from build123d import *

# Parameters (mm, degrees)
SKETCH1_W            = 170
SKETCH1_H            = 72
BOSS_EXTRUDE1_DEPTH  = 5
SKETCH2_R            = 5.5
SKETCH2_R_2          = 3.025
BOSS_EXTRUDE2_DEPTH  = 5
BOSS_EXTRUDE3_DEPTH  = 5
FILLET1_R            = 6
M4_CLEARANCE_HOLE1_D = 4.5


with BuildPart() as part:
    # Sketch1 → Boss-Extrude1 (new body)
    with BuildSketch(Plane.XY):
        Rectangle(SKETCH1_W, SKETCH1_H)
    extrude(amount=BOSS_EXTRUDE1_DEPTH)

    # Sketch2 → Boss-Extrude2 (add)
    # profile 1 of 6: a face of its own
    with BuildSketch(Plane.XY.offset(5)):
        with Locations((65, 25)):
            Circle(SKETCH2_R)
        with Locations((65, 25)):
            Circle(SKETCH2_R_2, mode=Mode.SUBTRACT)
    # profile 2 of 6: a face of its own
    with BuildSketch(Plane.XY.offset(5)):
        with Locations((8.25, 25)):
            Circle(SKETCH2_R)
        with Locations((8.25, 25)):
            Circle(SKETCH2_R_2, mode=Mode.SUBTRACT)
    # profile 3 of 6: a face of its own
    with BuildSketch(Plane.XY.offset(5)):
        with Locations((-65, 25)):
            Circle(SKETCH2_R)
        with Locations((-65, 25)):
            Circle(SKETCH2_R_2, mode=Mode.SUBTRACT)
    # profile 4 of 6: a face of its own
    with BuildSketch(Plane.XY.offset(5)):
        with Locations((-65, -25)):
            Circle(SKETCH2_R)
        with Locations((-65, -25)):
            Circle(SKETCH2_R_2, mode=Mode.SUBTRACT)
    # profile 5 of 6: a face of its own
    with BuildSketch(Plane.XY.offset(5)):
        with Locations((8.25, -25)):
            Circle(SKETCH2_R)
        with Locations((8.25, -25)):
            Circle(SKETCH2_R_2, mode=Mode.SUBTRACT)
    # profile 6 of 6: a face of its own
    with BuildSketch(Plane.XY.offset(5)):
        with Locations((65, -25)):
            Circle(SKETCH2_R)
        with Locations((65, -25)):
            Circle(SKETCH2_R_2, mode=Mode.SUBTRACT)
    extrude(amount=BOSS_EXTRUDE2_DEPTH)

    # Sketch3 → Boss-Extrude3 (add)
    with BuildSketch(Plane.XY.offset(5)):
        Polygon((-65, 51), (-85, 36), (-85, 51), align=None)
        Polygon((-65, 51), (-85, 36), (-65, 36), align=None)
        Polygon((65, -51), (85, -36), (65, -36), align=None)
        Polygon((85, -36), (85, -51), (65, -51), align=None)
    extrude(amount=-BOSS_EXTRUDE3_DEPTH)

    # Fillet1
    fillet1_edges = [part.edges().sort_by_distance(p)[0] for p in [
        (-85, 51, 2.5),
        (-65, 51, 2.5),
        (-65, 36, 2.5),
        (65, -51, 2.5),
        (65, -36, 2.5),
        (85, -51, 2.5),
        (-85, -36, 2.5),
        (85, 36, 2.5),
    ]]
    fillet(fillet1_edges, radius=FILLET1_R)

    # M4 Clearance Hole1 (through all)
    with Locations(Plane.XY.offset(5)):
        with Locations((-75, 43.5), (75, -43.5)):
            Hole(M4_CLEARANCE_HOLE1_D / 2)


solid = part.part
Part model, mm, in its own coordinate system. A direction names the side the tool comes from. Coordinates: 2 decimals unless noted, no trailing zeros. Write each loop counter-clockwise with the first axis right and the second up, starting at its lowest first coordinate (ties: lowest second). Pieces come first, ordered by that corner, then holes. Notation, with made-up numbers: (-26, 40.5) - (-10, 40.5) arc R18 cw to (-10, 64.5) - close; hole circle Ø9 at (49.25, -6). An arc over 180 degrees is marked (long way). Put each result on its own line as item: value.
1. Probe line 1 along Y through (x, z) = (8.25, 6.1) (3 decimals); line 2 along X through (y, z) = (30, 7); line 3 along Y through (x, z) = (67, 6.75). List the from-to ranges inside material, lowest first. Write a range as [from, to].
Final values:
line 1: y = [-30.5, -28.025], [-21.975, -19.5], [19.5, 21.975], [28.025, 30.5]
line 2: x = [-67.29, -62.71], [5.96, 10.54], [62.71, 67.29]
line 3: y = [-30.12, -27.27], [-22.73, -19.88], [19.88, 22.73], [27.27, 30.12]
2. Band-saw the part on C-C (x = 75). Write the cut outline in (y, z).
Final values:
outline: (-51, 0) - (-45.75, 0) - (-45.75, 5) - (-51, 5) - close; (-41.25, 0) - (36, 0) - (36, 5) - (-41.25, 5) - close
3. Band-saw the part on B-B (x = 8.25). Write the cut outline in (y, z) (3 decimals), then the cut area to 4 significant figures.
Final values:
outline: (-36, 0) - (36, 0) - (36, 5) - (30.5, 5) - (30.5, 10) - (28.025, 10) - (28.025, 5) - (21.975, 5) - (21.975, 10) - (19.5, 10) - (19.5, 5) - (-19.5, 5) - (-19.5, 10) - (-21.975, 10) - (-21.975, 5) - (-28.025, 5) - (-28.025, 10) - (-30.5, 10) - (-30.5, 5) - (-36, 5) - close
area: 409.5 mm²
4. Flat gauge pins, fed straight in: pin 1 Ø5.5 at (x, z) = (-4, 1.5) entering from +Y; pin 2 Ø2.5 at (x, z) = (-16, 2.5) entering from -Y; pin 3 Ø3 at (x, y) = (-65.5, -24.5) entering from +Z; pin 4 Ø5 at (x, y) = (-30.5, -39) entering from -Z. Where does each tip first touch, or does it go through?
Final values:
pin 1: stops at y = 36
pin 2: stops at y = -36
pin 3: stops at z = 5
pin 4: passes through
5. Band-saw the part on A-A (z = 7). Give the number of separate pieces and of enclosed holes in the cut face, then the cut area to 3 significant figures.
Final values:
separate pieces: 6
enclosed holes: 6
area: 398 mm²
6. Band-saw the part on D-D (y = 25). Write the cut outline in (x, z) (3 decimals), then the cut area to 3 significant figures.
Final values:
outline: (-85, 0) - (85, 0) - (85, 5) - (70.5, 5) - (70.5, 10) - (68.025, 10) - (68.025, 5) - (61.975, 5) - (61.975, 10) - (59.5, 10) - (59.5, 5) - (13.75, 5) - (13.75, 10) - (11.275, 10) - (11.275, 5) - (5.225, 5) - (5.225, 10) - (2.75, 10) - (2.75, 5) - (-59.5, 5) - (-59.5, 10) - (-61.975, 10) - (-61.975, 5) - (-68.025, 5) - (-68.025, 10) - (-70.5, 10) - (-70.5, 5) - (-85, 5) - close
area: 924 mm²
7. 3-axis set-ups, long thin cutter, end or side, ignore diameter. For faces 1 (the cylindrical face through (7.86, -22, 7.46)), 2 (the flat face through (-11, -36, 2)), 3 (the flat face through (-85, 7, 3)): which of +Z, -Z, +X, -X, +Y, -Y reach the whole face in a straight line?
Final values:
face 1: +Z
face 2: +Z, -Z, -X, -Y
face 3: +Z, -Z, -X, +Y, -Y
